For this review, take the finished solid that the model builds, in its own axes (mm). A direction names the side the tool comes from. Coordinates: 2 decimals unless noted, no trailing zeros. Order: outer loops, then holes, each group sorted by start corner. A loop starts at its lowest first (then second) coordinate and runs counter-clockwise, first axis right, second up. Notation, with made-up numbers: (-21.5, 77.5) - (1.5, 77.5) arc R16 cw to (1.5, 94.5) - close; hole circle Ø5 at (59, 8). An arc over 180 degrees is marked (long way). One line per item, written item: value. Start each with the question number.
(1) Consider section C-C on z = 16. Write out the cut boundary in (x, y), then the cut area to 3 significant figures.
(2) To check wall thickness, follow line 1 along Z through (x, y) = (-56.5, -0.65); line 2 along Z through (x, y) = (-57.5, -1.65); line 3 along X through (y, z) = (-2.7, 18.5). State the ranges of each line that lie inside material, in increasing order.
(3) For faces 4 (the flat face through (-53.137, -1, 19)), 5 (the flat face through (36.863, -1, 1)), 6 (the flat face through (42, -1, 15)), list the 3-axis set-ups (+Z, -Z, +X, -X, +Y, -Y) from which the entire face can be reached by the end or side of a thin tool; tool diameter is ignored.
(4) Consider section D-D on z = 3.75. Write out the cut boundary in (x, y), then the cut area to 3 significant figures.
(5) Clearance check with flat-ended pins moving along their axes: pin 1 (0.9 mm diameter, centred on x = -58, y = -1.5, fed in from +Z); pin 2 (1 mm diameter, centred on y = -2, z = 1.5, fed in from +X); pin 3 (0.6 mm diameter, centred on y = -1, z = 19, fed in from -X). State where each tip first meets the part, or that it passes through.
(6) Mouldability with a two-part tool opening along X and no side actions: class faces 1 (the flat face through (-58, -1, 15)), 2 (the cylindrical face through (-59.236, -1.479, 10.048)), 3 (the cylindrical face through (-53.993, -1.521, 15.902)) as released by +X, released by -X, zero draft, split by the parting line, or undercut.
(7) Consider section B-B on y = -1.5. Write out the cut boundary in (x, z), then the cut area to 3 significant figures.
(8) Consider section A-A on z = 10. Write out the cut boundary in (x, y), then the cut area to 3 significant figures.
```python
from build123d import *

# Parameters (mm, degrees)
F0_R     = 1.1
F1_DEPTH = 3
F2_R     = 3


with BuildPart() as f1:
    # F0 (on Front) → F1 (new body)
    with BuildSketch(Plane.XZ):
        with BuildLine():
            Line((36.86291, 20), (-53.13709, 20))
            Line((-53.13709, 20), (-53.13709, 15))
            Line((-53.13709, 15), (-63.13709, 15))
            Line((-63.13709, 15), (-63.13709, 5))
            Line((-63.13709, 5), (-53.13709, 5))
            Line((-53.13709, 5), (-53.13709, 0))
            Line((-53.13709, 0), (36.86291, 0))
            Line((36.86291, 0), (36.86291, 2))
            ThreePointArc((36.86291, 2), (37.74159, 4.12132), (39.86291, 5))
            Line((39.86291, 5), (46.86291, 5))
            Line((46.86291, 5), (46.86291, 15))
            Line((46.86291, 15), (39.86291, 15))
            ThreePointArc((39.86291, 15), (37.74159, 15.87868), (36.86291, 18))
            Line((36.86291, 18), (36.86291, 20))
        make_face()
        with Locations((-58.13709, 10)):
            Circle(F0_R, mode=Mode.SUBTRACT)
        with Locations((41.86291, 10)):
            Circle(F0_R, mode=Mode.SUBTRACT)
    extrude(amount=F1_DEPTH)

    # F2
    f2_edges = [f1.edges().sort_by_distance(p)[0] for p in [
        (-53.13709, -1.5, 15),
        (-53.13709, -1.5, 5),
        (-63.13709, -1.5, 15),
        (-63.13709, -1.5, 5),
        (46.86291, -1.5, 5),
        (46.86291, -1.5, 15),
    ]]
    fillet(f2_edges, radius=F2_R)


solid = f1.part
```
Geometry check:
1. outline: (-53.9, -3) - (37.63, -3) - (37.63, 0) - (-53.9, 0) - close
1. area: 275 mm^2
2. line 1: z = 5 to 15
2. line 2: z = 5 to 9.1, 10.9 to 15
2. line 3: x = -53.14 to 36.86
3. face 4: +Z, -X, +Y, -Y
3. face 5: -Z, +X, +Y, -Y
3. face 6: +Z, +X, +Y, -Y
4. outline: (-53.7, -3) - (37.43, -3) - (37.43, 0) - (-53.7, 0) - close
4. area: 273 mm^2
5. pin 1: stops at z = 15
5. pin 2: stops at x = 36.86
5. pin 3: stops at x = -53.14
6. face 1: zero draft
6. face 2: undercut
6. face 3: released by -X
7. outline: (-63.14, 8) arc R3 ccw to (-60.14, 5) - (-56.14, 5) arc R3 cw to (-53.14, 2) - (-53.14, 0) - (36.86, 0) - (36.86, 2) arc R3 cw to (39.86, 5) - (43.86, 5) arc R3 ccw to (46.86, 8) - (46.86, 12) arc R3 ccw to (43.86, 15) - (39.86, 15) arc R3 cw to (36.86, 18) - (36.86, 20) - (-53.14, 20) - (-53.14, 18) arc R3 cw to (-56.14, 15) - (-60.14, 15) arc R3 ccw to (-63.14, 12) - close; hole circle Ø2.2 at (-58.14, 10); hole circle Ø2.2 at (41.86, 10)
7. area: 1,990 mm^2
8. outline: (-63.14, -3) - (-59.24, -3) - (-59.24, 0) - (-63.14, 0) - close; (-57.04, -3) - (40.76, -3) - (40.76, 0) - (-57.04, 0) - close; (42.96, -3) - (46.86, -3) - (46.86, 0) - (42.96, 0) - close
8. area: 317 mm^2
